```python
from build123d import *

# Parameters (mm, degrees)
SKETCH1_R           = 27.889608224
SKETCH1_R_2         = 3.25
SKETCH1_R_3         = 11
SKETCH1_R_4         = 3.5
BOSS_EXTRUDE1_DEPTH = 3
SKETCH1_5_R         = 11
SKETCH1_5_R_2       = 3.5
BOSS_EXTRUDE2_DEPTH = 1
BOSS_EXTRUDE3_DEPTH = 6
CHAMFER1_SIZE       = 4
SKETCH3_R           = 1.5
CUT_EXTRUDE1_DEPTH  = 6
CIRPATTERN1_COUNT   = 4


with BuildPart() as part:
    # Sketch1 → Boss-Extrude1 (new body)
    with BuildSketch(Plane(origin=(0, 0, 0), x_dir=(1, 0, 0), z_dir=(0, 1, 0))):
        Circle(SKETCH1_R)
        with Locations((-15.55, 15.55)):
            Circle(SKETCH1_R_2, mode=Mode.SUBTRACT)
        with Locations((-15.55, -15.55)):
            Circle(SKETCH1_R_2, mode=Mode.SUBTRACT)
        with Locations((15.55, -15.55)):
            Circle(SKETCH1_R_2, mode=Mode.SUBTRACT)
        with Locations((15.55, 15.55)):
            Circle(SKETCH1_R_2, mode=Mode.SUBTRACT)
        Circle(SKETCH1_R_3, mode=Mode.SUBTRACT)
        Circle(SKETCH1_R_3)
        Circle(SKETCH1_R_4, mode=Mode.SUBTRACT)
    extrude(amount=-BOSS_EXTRUDE1_DEPTH)

    # Sketch1_5 → Boss-Extrude2 (add)
    with BuildSketch(Plane(origin=(0, 0, 0), x_dir=(1, 0, 0), z_dir=(0, 1, 0))):
        Circle(SKETCH1_5_R)
        Circle(SKETCH1_5_R_2, mode=Mode.SUBTRACT)
    extrude(amount=BOSS_EXTRUDE2_DEPTH)

    # Sketch2 → Boss-Extrude3 (add)
    with BuildSketch(Plane.XZ.offset(3)):
        with BuildLine():
            Line((-19.607997757, -3), (-7.607997757, -3))
            ThreePointArc((-7.607997757, -3), (-8.178118969, 0), (-7.607997757, 3))
            Line((-7.607997757, 3), (-19.607997757, 3))
            Line((-19.607997757, 3), (-19.607997757, -3))
        make_face()
        with BuildLine():
            Line((-3, 19.607997757), (3, 19.607997757))
            Line((3, 19.607997757), (3, 7.607997757))
            ThreePointArc((3, 7.607997757), (0, 8.178118969), (-3, 7.607997757))
            Line((-3, 7.607997757), (-3, 19.607997757))
        make_face()
        with BuildLine():
            Line((19.607997757, -3), (7.607997757, -3))
            ThreePointArc((7.607997757, -3), (8.178118969, 0), (7.607997757, 3))
            Line((7.607997757, 3), (19.607997757, 3))
            Line((19.607997757, 3), (19.607997757, -3))
        make_face()
        with BuildLine():
            Line((-3, -19.607997757), (3, -19.607997757))
            Line((3, -19.607997757), (3, -7.607997757))
            ThreePointArc((3, -7.607997757), (0, -8.178118969), (-3, -7.607997757))
            Line((-3, -7.607997757), (-3, -19.607997757))
        make_face()
    extrude(amount=BOSS_EXTRUDE3_DEPTH)

    # Chamfer1
    chamfer1_edges = [part.edges().sort_by_distance(p)[0] for p in [
        (-8.178118969, -9, 0),
        (0, -9, 8.178118969),
        (8.178118969, -9, 0),
        (0, -9, -8.178118969),
    ]]
    chamfer(chamfer1_edges, length=CHAMFER1_SIZE)

    # Sketch3 → Cut-Extrude1 (cut)
    with BuildSketch(Plane.ZY.offset(19.607997757)):
        with Locations((0, -6)):
            Circle(SKETCH3_R)
    cut_extrude1 = extrude(amount=-CUT_EXTRUDE1_DEPTH, mode=Mode.SUBTRACT)

    # CirPattern1: Cut-Extrude1 ×4 about axis
    cirpattern1_axis = Axis((0, 0, 0), (0, 1, 0))
    for i in range(1, CIRPATTERN1_COUNT):
        add(cut_extrude1.rotate(cirpattern1_axis, i * 360 / CIRPATTERN1_COUNT), mode=Mode.SUBTRACT)


solid = part.part
```
Could you check a few things on this model? Use its own coordinates, in mm. A direction names the side the tool comes from. Give positions to 0.01 mm unless a question says otherwise; leave off trailing zeros. Order: outer loops, then holes, each group sorted by start corner. A loop starts at its lowest first (then second) coordinate and runs counter-clockwise, first axis right, second up.
Q1. Suppose I cut it at D-D, the plane y = -1.25. Write out the boundary of the cut face in (x, z).
Q2. If I drill on line 1 along Z through (x, y) = (15.55, -1.3); line 2 along Z through (x, y) = (0, -1.25); line 3 along Y through (x, z) = (0, 18.05), over which ranges is the centre line in solid material (lowest first)?
Q3. I'm going to push flat-ended pins straight in: P1, Ø3, axis at y = -5.5, z = 0.5, coming from the -X side; P2, Ø6, axis at x = -4.5, y = -1.5, coming from the +Z side; P3, Ø3, axis at x = -18, y = -2, coming from the +Z side; P4, Ø1.5, axis at y = -4.5, z = -4, coming from the +X side. Where does each tip first touch, or does it pass through?
Q4. Suppose I cut it at B-B, the plane x = 15.55. Write out the boundary of the cut face in (y, z), and give its area (3 significant figures).
Q5. We'd pull the mould along X, two halves only. Please class faces 5 (the cylindrical face through (16.65, -7.464, 0.325)), 6 (the cylindrical face through (-2.38, 0.49, 10.74)), 7 (the flat face through (0, -6, -13.608)): +X half, -X half, draft (parallel to the pull), parting line (faces both ways), or undercut.
Q6. For faces 1 (the flat face through (-14, -6, -3)), 2 (the flat face through (3, -6, 14)), 3 (the flat face through (13.608, -6, 0)), 4 (the conical face through (10.21, -7.03, -0.05)), which set-ups out of +Z, -Z, +X, -X, +Y, -Y let a thin tool reach every point of the face, with its end or its side?
Q7. Suppose I cut it at A-A, the plane z = 17. Write out the boundary of the cut face in (x, y), and give its area (3 significant figures).
Solution:
1. outline: circle Ø55.78 at (0, 0); hole circle Ø6.5 at (-15.55, -15.55); hole circle Ø6.5 at (-15.55, 15.55); hole circle Ø7 at (0, 0); hole circle Ø6.5 at (15.55, -15.55); hole circle Ø6.5 at (15.55, 15.55)
2. line 1: z = -23.15 to -18.8, -12.3 to 12.3, 18.8 to 23.15
2. line 2: z = -27.89 to -3.5, 3.5 to 27.89
2. line 3: y = -9 to -7.5, -4.5 to 0
3. P1: stops at x = -19.61
3. P2: stops at z = 27.85
3. P3: stops at z = 22.49
3. P4: passes through
4. outline: (-9, -3) - (-3, -3) - (-3, -12.3) - (0, -12.3) - (0, 12.3) - (-3, 12.3) - (-3, 3) - (-9, 3) - close; (-3, -23.15) - (0, -23.15) - (0, -18.8) - (-3, -18.8) - close; (-3, 18.8) - (0, 18.8) - (0, 23.15) - (-3, 23.15) - close; hole circle Ø3 at (-6, 0)
4. area: 129 mm2
5. face 5: draft
5. face 6: parting line
5. face 7: undercut
6. face 1: -Z, +X, -X, -Y
6. face 2: +Z, -Z, +X, -Y
6. face 3: +X
6. face 4: -Y
7. outline: (-22.11, -3) - (-18.46, -3) - (-18.46, 0) - (-22.11, 0) - close; (-12.64, -3) - (-3, -3) - (-3, -9) - (3, -9) - (3, -3) - (12.64, -3) - (12.64, 0) - (-12.64, 0) - close; (18.46, -3) - (22.11, -3) - (22.11, 0) - (18.46, 0) - close; hole circle Ø3 at (0, -6)
7. area: 127 mm2
